Verification items for the finished model (mm, model axes). Face numbers are marked on the shaded views. A direction names the side the tool comes from. Round coordinates to 2 decimals unless told otherwise and drop trailing zeros. Order: outer loops, then holes, each group sorted by start corner. A loop starts at its lowest first (then second) coordinate and runs counter-clockwise, first axis right, second up. Notation, with made-up numbers: M -19,-2 L 36,-2 A24 ccw 36,30 Z; hole C -18.75,0.5 d10. An arc over 180 degrees is marked long. Return JSON: item names as keys, results as strings. Group by question number.
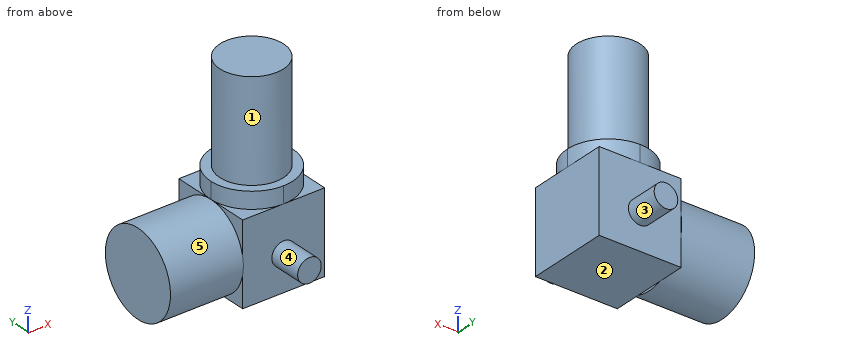
from build123d import *

# Parameters (mm, degrees)
SKETCH1_W           = 25.146
SKETCH1_H           = 25.146
BOSS_EXTRUDE1_DEPTH = 24.892
BOSS_EXTRUDE2_DEPTH = 5.08
SKETCH3_R           = 9.779
BOSS_EXTRUDE3_DEPTH = 30.48
SKETCH4_R           = 12.827
BOSS_EXTRUDE4_DEPTH = 22.352
SKETCH5_R           = 3.6195
BOSS_EXTRUDE5_DEPTH = 10.16
BOSS_EXTRUDE6_START = 10.16
SKETCH6_R           = 3.6195
BOSS_EXTRUDE6_DEPTH = 10.16


with BuildPart() as part:
    # Sketch1 → Boss-Extrude1 (new body)
    with BuildSketch(Plane.XY):
        with Locations((-15.408088235, -0.246529412)):
            Rectangle(SKETCH1_W, SKETCH1_H)
    extrude(amount=BOSS_EXTRUDE1_DEPTH)

    # Sketch2 → Boss-Extrude2 (add)
    with BuildSketch(Plane.XY.offset(24.892)):
        with BuildLine():
            ThreePointArc((-2.835088235, -0.246529412), (-6.517634675, 8.643924148), (-15.408088235, 12.326470588))
            Line((-15.408088235, 12.326470588), (-15.408088235, -0.246529412))
            Line((-15.408088235, -0.246529412), (-2.835088235, -0.246529412))
        make_face()
        with BuildLine():
            Line((-15.408088235, -0.246529412), (-15.408088235, 12.326470588))
            ThreePointArc((-15.408088235, 12.326470588), (-24.298541795, 8.643924148), (-27.981088235, -0.246529412))
            Line((-27.981088235, -0.246529412), (-15.408088235, -0.246529412))
        make_face()
        with BuildLine():
            Line((-2.835088235, -0.246529412), (-15.408088235, -0.246529412))
            Line((-15.408088235, -0.246529412), (-15.408088235, -12.819529412))
            ThreePointArc((-15.408088235, -12.819529412), (-6.517634675, -9.136982972), (-2.835088235, -0.246529412))
        make_face()
        with BuildLine():
            Line((-15.408088235, -12.819529412), (-15.408088235, -0.246529412))
            Line((-15.408088235, -0.246529412), (-27.981088235, -0.246529412))
            ThreePointArc((-27.981088235, -0.246529412), (-24.298541795, -9.136982972), (-15.408088235, -12.819529412))
        make_face()
        with BuildLine():
            ThreePointArc((-2.835088235, -0.246529412), (-6.517634675, 8.643924148), (-15.408088235, 12.326470588))
            Line((-15.408088235, 12.326470588), (-15.408088235, -0.246529412))
            Line((-15.408088235, -0.246529412), (-2.835088235, -0.246529412))
        make_face()
        with BuildLine():
            Line((-15.408088235, -0.246529412), (-15.408088235, 12.326470588))
            ThreePointArc((-15.408088235, 12.326470588), (-24.298541795, 8.643924148), (-27.981088235, -0.246529412))
            Line((-27.981088235, -0.246529412), (-15.408088235, -0.246529412))
        make_face()
        with BuildLine():
            Line((-2.835088235, -0.246529412), (-15.408088235, -0.246529412))
            Line((-15.408088235, -0.246529412), (-15.408088235, -12.819529412))
            ThreePointArc((-15.408088235, -12.819529412), (-6.517634675, -9.136982972), (-2.835088235, -0.246529412))
        make_face()
        with BuildLine():
            Line((-15.408088235, -12.819529412), (-15.408088235, -0.246529412))
            Line((-15.408088235, -0.246529412), (-27.981088235, -0.246529412))
            ThreePointArc((-27.981088235, -0.246529412), (-24.298541795, -9.136982972), (-15.408088235, -12.819529412))
        make_face()
        with BuildLine():
            ThreePointArc((-2.835088235, -0.246529412), (-6.517634675, 8.643924148), (-15.408088235, 12.326470588))
            Line((-15.408088235, 12.326470588), (-15.408088235, -0.246529412))
            Line((-15.408088235, -0.246529412), (-2.835088235, -0.246529412))
        make_face()
        with BuildLine():
            Line((-15.408088235, -0.246529412), (-15.408088235, 12.326470588))
            ThreePointArc((-15.408088235, 12.326470588), (-24.298541795, 8.643924148), (-27.981088235, -0.246529412))
            Line((-27.981088235, -0.246529412), (-15.408088235, -0.246529412))
        make_face()
        with BuildLine():
            Line((-2.835088235, -0.246529412), (-15.408088235, -0.246529412))
            Line((-15.408088235, -0.246529412), (-15.408088235, -12.819529412))
            ThreePointArc((-15.408088235, -12.819529412), (-6.517634675, -9.136982972), (-2.835088235, -0.246529412))
        make_face()
        with BuildLine():
            Line((-15.408088235, -12.819529412), (-15.408088235, -0.246529412))
            Line((-15.408088235, -0.246529412), (-27.981088235, -0.246529412))
            ThreePointArc((-27.981088235, -0.246529412), (-24.298541795, -9.136982972), (-15.408088235, -12.819529412))
        make_face()
        with BuildLine():
            ThreePointArc((-2.835088235, -0.246529412), (-6.517634675, 8.643924148), (-15.408088235, 12.326470588))
            Line((-15.408088235, 12.326470588), (-15.408088235, -0.246529412))
            Line((-15.408088235, -0.246529412), (-2.835088235, -0.246529412))
        make_face()
        with BuildLine():
            Line((-15.408088235, -0.246529412), (-15.408088235, 12.326470588))
            ThreePointArc((-15.408088235, 12.326470588), (-24.298541795, 8.643924148), (-27.981088235, -0.246529412))
            Line((-27.981088235, -0.246529412), (-15.408088235, -0.246529412))
        make_face()
        with BuildLine():
            Line((-2.835088235, -0.246529412), (-15.408088235, -0.246529412))
            Line((-15.408088235, -0.246529412), (-15.408088235, -12.819529412))
            ThreePointArc((-15.408088235, -12.819529412), (-6.517634675, -9.136982972), (-2.835088235, -0.246529412))
        make_face()
        with BuildLine():
            Line((-15.408088235, -12.819529412), (-15.408088235, -0.246529412))
            Line((-15.408088235, -0.246529412), (-27.981088235, -0.246529412))
            ThreePointArc((-27.981088235, -0.246529412), (-24.298541795, -9.136982972), (-15.408088235, -12.819529412))
        make_face()
    extrude(amount=BOSS_EXTRUDE2_DEPTH)

    # Sketch3 → Boss-Extrude3 (add)
    with BuildSketch(Plane.XY.offset(29.972)):
        with Locations(Location((-15.408088235, -0.246529412, 0), (0, 0, 180))):
            Circle(SKETCH3_R)
    extrude(amount=BOSS_EXTRUDE3_DEPTH)

    # Sketch4 → Boss-Extrude4 (add)
    with BuildSketch(Plane.ZY.offset(27.981088235)):
        with Locations((12.065, -0.246529412)):
            Circle(SKETCH4_R)
    extrude(amount=BOSS_EXTRUDE4_DEPTH)

    # Sketch5 → Boss-Extrude5 (add)
    with BuildSketch(Plane.XZ.offset(12.819529412)):
        with Locations(Location((-15.408088235, 10.922, 0), (0, 0, 90))):
            Circle(SKETCH5_R)
    extrude(amount=BOSS_EXTRUDE5_DEPTH)

    # Sketch6 → Boss-Extrude6 (add)
    with BuildSketch(Plane(origin=(0, 12.326470588, 0), x_dir=(1, 0, 0), z_dir=(0, 1, 0)).offset(BOSS_EXTRUDE6_START)):
        with Locations(Location((-15.408088235, -10.922, 0), (0, 0, 270))):
            Circle(SKETCH6_R)
    extrude(amount=-BOSS_EXTRUDE6_DEPTH)


solid = part.part
1. Access from +Z, -Z, +X, -X, +Y, -Y to the whole of each face (thin tool, end or side, straight path). Record for the marked faces 1, 2, 3, 4 and 5.
2. Cross-section at B-B (y = 3). Enter the section's corners in (x, z).
3. Thickness scan on line 1 along Z through (x, y) = (-20, 4.5); line 2 along Y through (x, z) = (-11, 7); line 3 along Y through (x, z) = (-36.5, 12). Record the ranges inside material, lowest first. Write a range as from..to.
4. Cross-section at A-A (x = -14). Enter the section's corners in (y, z), plus the area to 3 significant figures.
5. Cross-section at C-C (z = 39). Enter the section's corners in (x, y).
6. Cross-section at D-D (x = -30). Enter the section's corners in (y, z) (3 decimals).
7. Go/stop test with flat-tipped pins: pin 1 (8 mm diameter, centred on x = -45, y = 9, fed in from -Z); pin 2 (2 mm diameter, centred on x = -40.5, y = 1.5, fed in from +Z); pin 3 (20 mm diameter, centred on x = -14.5, y = -6, fed in from -Z). Record where each tip stops, or that it passes through.
Computed:
{
 "1": {"face 1": "+Z", "face 2": "-Z, +X, +Y, -Y", "face 3": "+Y", "face 4": "-Y", "face 5": "-X"},
 "2": {"outline": "M -50.33,-0.34 L -27.98,-0.34 L -27.98,0 L -2.84,0 L -2.84,24.89 L -3.26,24.89 L -3.26,29.97 L -6.18,29.97 L -6.18,60.45 L -24.63,60.45 L -24.63,29.97 L -27.55,29.97 L -27.55,24.89 L -27.98,24.89 L -27.98,24.47 L -50.33,24.47 Z"},
 "3": {"line 1": "z = 0..60.45", "line 2": "y = -12.82..12.33", "line 3": "y = -13.07..12.58"},
 "4": {"outline": "M -22.98,7.59 L -12.82,7.59 L -12.82,0 L 12.33,0 L 12.33,7.59 L 22.49,7.59 L 22.49,14.26 L 12.33,14.26 L 12.33,24.89 L 12.25,24.89 L 12.25,29.97 L 9.43,29.97 L 9.43,60.45 L -9.92,60.45 L -9.92,29.97 L -12.74,29.97 L -12.74,24.89 L -12.82,24.89 L -12.82,14.26 L -22.98,14.26 Z", "area": "1,480 mm²"},
 "5": {"outline": "C -15.41,-0.25 d19.56"},
 "6": {"outline": "C -0.247,12.065 d25.654"},
 "7": {"pin 1": "stops at z = 0.36", "pin 2": "stops at z = 24.87", "pin 3": "stops at z = 0"}
}
